from build123d import *

# Parameters (mm, degrees)
F1_DEPTH = 3
F2_R     = 5.75
F2_R_2   = 1.7
F3_DEPTH = 3
F4_R     = 1.5
F5_R     = 5
F6_R     = 2
F7_R     = 2


with BuildPart() as f1:
    # F0 (on Top) → F1 (new body)
    with BuildSketch(Plane.XY):
        Polygon((50.8348240464, 59.6463644877), (-29.1651759536, -20.3536355123), (50.8348240464, -20.3536355123), align=None)
    extrude(amount=F1_DEPTH)

    # F2 (on face) → F3 (cut, through all)
    with BuildSketch(Plane.XY.offset(3)):
        Polygon((0.734318983, -0.3536355123), (30.8348240464, -0.3536355123), (30.8348240464, 29.7468695511), align=None)
        with Locations((40.8348240464, -10.3536355123)):
            Circle(F2_R)
        with Locations((15.8348240464, -10.3536355123)):
            Circle(F2_R_2)
        with Locations((-4.1651759536, -10.3536355123)):
            Circle(F2_R_2)
        with Locations((40.8348240464, 14.6463644877)):
            Circle(F2_R_2)
        with Locations((40.8348240464, 34.6463644877)):
            Circle(F2_R_2)
    extrude(amount=-F3_DEPTH, mode=Mode.SUBTRACT)

    # F4
    f4_edges = [f1.edges().sort_by_distance(p)[0] for p in [
        (0.734319, -0.353636, 1.5),
        (30.834824, -0.353636, 1.5),
        (30.834824, 29.74687, 1.5),
    ]]
    fillet(f4_edges, radius=F4_R)

    # F5
    f5_edges = [f1.edges().sort_by_distance(p)[0] for p in [
        (-29.165176, -20.353636, 1.5),
        (50.834824, -20.353636, 1.5),
        (50.834824, 59.646364, 1.5),
    ]]
    fillet(f5_edges, radius=F5_R)

    # F6
    f6_edges = [f1.edges().sort_by_distance(p)[0] for p in [
        (14.370358, -20.353636, 3),
        (49.370358, -18.889169, 3),
        (50.834824, 16.110831, 3),
        (-21.713506, -17.267053, 3),
        (10.834824, 19.646364, 3),
        (47.748241, 52.194694, 3),
    ]]
    fillet(f6_edges, radius=F6_R)

    # F7
    f7_edges = [f1.edges().sort_by_distance(p)[0] for p in [
        (16.845232, -0.353636, 3),
        (30.834824, 13.635957, 3),
        (15.784572, 14.696617, 3),
        (30.395484, 0.085704, 3),
        (2.96982, 0.572339, 3),
        (29.908849, 27.511369, 3),
    ]]
    fillet(f7_edges, radius=F7_R)


solid = f1.part
Source: CAD feature listing. Evaluate the final solid. Frame: model axes, mm. A direction names the side the tool comes from. Give positions to 0.01 mm unless a question says otherwise; leave off trailing zeros. Order: outer loops, then holes, each group sorted by start corner. A loop starts at its lowest first (then second) coordinate and runs counter-clockwise, first axis right, second up. Notation, with made-up numbers: (-31, -30) -> (21, -30) arc R6 ccw to (21, -23) -> close; hole circle Ø7 at (-33, 78.5). An arc over 180 degrees is marked (long way). Use a Markdown table: item, result.
1) Section query A-A, the plane z = 2. Return the cut outline in (x, y).
Answer list:
| item | result |
|---|---|
| outline | (-20.44, -12.01) arc R4.73 ccw to (-17.09, -20.09) -> (45.83, -20.09) arc R4.73 ccw to (50.57, -15.35) -> (50.57, 47.58) arc R4.73 ccw to (42.49, 50.92) -> close; hole circle Ø3.4 at (-4.17, -10.35); hole (3.11, 2.4) arc R1.77 ccw to (4.36, -0.62) -> (29.33, -0.62) arc R1.77 ccw to (31.1, 1.15) -> (31.1, 26.13) arc R1.77 ccw to (28.08, 27.38) -> close; hole circle Ø3.4 at (15.83, -10.35); hole circle Ø11.5 at (40.83, -10.35); hole circle Ø3.4 at (40.83, 14.65); hole circle Ø3.4 at (40.83, 34.65) |
2) Ray query, line 1 along Y through (x, z) = (16, 2.05); line 2 along X through (y, z) = (16, 0.7); line 3 along X through (y, z) = (-9, 2.3). Return the intervals inside material, ascending. Write a range as [from, to].
Answer list:
| item | result |
|---|---|
| line 1 | [-20.06, -12.05], [-8.66, -0.65], [15.33, 24.39] |
| line 2 | [7.19, 17.09], [30.83, 39.81], [41.86, 50.83] |
| line 3 | [-17.13, -5.19], [-3.14, 14.81], [16.86, 35.25], [46.42, 50.35] |
3) Reachability of faces 1 (the cylindrical face through (10.8, 18.8, 2.4)), 2 (the cylindrical face through (17.02, -0.955, 2.43)) from +Z, -Z, +X, -X, +Y, -Y: full face, straight path, thin tool, end or side. Return the list, or none.
Answer list:
| item | result |
|---|---|
| face 1 | +Z, -X, +Y |
| face 2 | +Z |
4) Mould query, pull axis X, two halves, no side actions, for faces 3 (the cylindrical face through (14.81, -19.78, 2.4)), 4 (the flat face through (15.96, 14.87, 0.51)), 5 (the cylindrical face through (47.672, 52.226, 0.507)). Classes: +X half, -X half, draft (parallel to the pull), parting line (faces both ways), or undercut.
Answer list:
| item | result |
|---|---|
| face 3 | draft |
| face 4 | undercut |
| face 5 | parting line |
5) Contact query for flat-ended pins moving along their axis: P1, Ø1.5, axis at x = 32.5, z = 1, coming from the +Y side; P2, Ø1, axis at y = -8.5, z = 2.5, coming from the -X side; P3, Ø0.8, axis at y = 10, z = 0.5, coming from the -X side. Output: stop coordinate, or through.
Answer list:
| item | result |
|---|---|
| P1 | y = 42.06 |
| P2 | x = -17.15 |
| P3 | x = 0.79 |
